CAD build for the part. Positions are in the model's coordinates, mm. Face numbers are marked on the shaded views. Give positions to 0.01 mm unless a question says otherwise; leave off trailing zeros. Order: outer loops, then holes, each group sorted by start corner. A loop starts at its lowest first (then second) coordinate and runs counter-clockwise, first axis right, second up. Notation, with made-up numbers: (-13, -14.75) -> (14, -14.75) arc R28 ccw to (14, 20.25) -> close; hole circle Ø8 at (52.5, 8.5). An arc over 180 degrees is marked (long way). Answer as CSV lines item,"result".
Autodesk Inventor part; units mm, degrees
ref_plane "YZ Plane" through (0, 0, 0) normal (1, 0, 0) x (0, 1, 0)
ref_plane "XZ Plane" through (0, 0, 0) normal (0, 1, 0) x (-1, 0, 0)
ref_plane "XY Plane" through (0, 0, 0) normal (0, 0, 1) x (1, 0, 0)
sketch "Sketch1" plane through (0, 0, 0) normal (0, 0, 1) x (1, 0, 0)
  line L0 (-16, -5) -> (16, -5)
  line L1 (16, -5) -> (16, 5)
  line L2 (16, 5) -> (-16, 5)
  line L3 (-16, 5) -> (-16, -5)
  line L4 (-16, -5) -> (16, 5) construction
  line L5 (16, -5) -> (-16, 5) construction
  point P0 (0, 0)
  dimension "d0" = 32
  dimension "d1" = 10
extrude "Plate1" add sketch "Sketch1" along normal blind 0.5
sketch "Sketch2" plane through (15.5, 5, 0) normal (1, 0, 0) x (0, 1, 0)
  line L0 (-10, 0) -> (0, 0)
  line L1 (0, 0) -> (0, 30)
  line L2 (0, 30) -> (-10, 30)
  line L3 (-10, 30) -> (-10, 0)
edge flange "Flange1" height 30 angle 90 thickness 0.5 bend radius 0.5 thickness toward (1, 0, 0) relief tear relief width 0.5 relief depth 0.25 edges at (16, 0, 0.5) wall of the first edge with corners at (15.5, -5, 0) (15.5, 5, 0) (15.5, 5, 30) (15.5, -5, 30)
bend "Bend1"
corner "Corner1"
sketch "Sketch4" plane through (0, 0, 0.5) normal (0, 0, 1) x (1, 0, 0)
  line L0 (-16, -5) -> (-16, 5)
  point P0 (0, 0)
  point P1 (-12, 0)
  point P2 (-2, 0)
  dimension "d13" = 4
  dimension "d14" = 14
hole "Hole1" at (-12, 0, 0.5) at (-2, 0, 0.5) direction (0, 0, -1) diameter 4 end through all
sketch "Sketch5" plane through (16, -5, 30) normal (1, 0, 0) x (0, 0, -1)
  line L0 (0, 0) -> (0, 10)
  point P0 (30, 5)
  point P1 (4, 5)
  point P2 (14, 5)
  dimension "d22" = 4
  dimension "d23" = 14
hole "Hole2" at (16, 0, 26) at (16, 0, 16) direction (-1, 0, 0) diameter 4 end through all
equation "\"d20\" = Thickness"
equation "\"d29\" = Thickness"
equation "\"d3\" = BendReliefWidth"
equation "\"d4\" = BendReliefDepth"
equation "\"d5\" = MinimumRemnant"
equation "\"d6\" = BendRadius"
equation "\"d9\" = BendRadius"
equation "\"d10\" = CornerReliefSize"
equation "\"d11\" = GapSize"
equation "\"d12\" = JacobiRadiusSize"
equation "\"BendRadius\" = Thickness"
equation "\"BendReliefWidth\" = Thickness"
equation "\"BendReliefDepth\" = 0.5 * Thickness"
equation "\"CornerReliefSize\" = 4 * Thickness"
equation "\"MinimumRemnant\" = 2 * Thickness"
equation "\"TransitionRadius\" = BendRadius"
equation "\"JacobiRadiusSize\" = BendRadius"
equation "\"GapSize\" = Thickness"
equation "\"d2\" = BendRadius"
properties part number "maker-beam-corner"
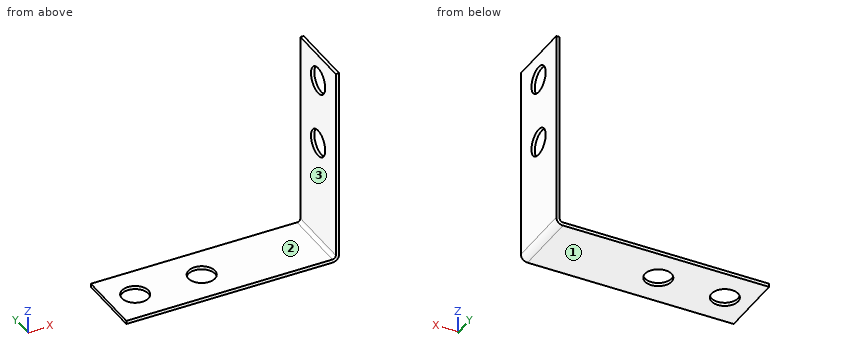
1) Band-saw the part on D-D, the plane y = -1.5. Write the cut outline in (x, z).
Data:
outline,"(-16, 0) -> (-13.32, 0) -> (-13.32, 0.5) -> (-16, 0.5) -> close; (-10.68, 0) -> (-3.32, 0) -> (-3.32, 0.5) -> (-10.68, 0.5) -> close; (-0.68, 0) -> (15, 0) arc R1 ccw to (16, 1) -> (16, 14.68) -> (15.5, 14.68) -> (15.5, 1) arc R0.5 cw to (15, 0.5) -> (-0.68, 0.5) -> close; (15.5, 17.32) -> (16, 17.32) -> (16, 24.68) -> (15.5, 24.68) -> close; (15.5, 27.32) -> (16, 27.32) -> (16, 30) -> (15.5, 30) -> close"
2) Band-saw the part on B-B, the plane z = 16. Write the cut outline in (x, y).
Data:
outline,"(15.5, -5) -> (16, -5) -> (16, -2) -> (15.5, -2) -> close; (15.5, 2) -> (16, 2) -> (16, 5) -> (15.5, 5) -> close"
3) Band-saw the part on A-A, the plane x = -12. Write the cut outline in (y, z).
Data:
outline,"(-5, 0) -> (-2, 0) -> (-2, 0.5) -> (-5, 0.5) -> close; (2, 0) -> (5, 0) -> (5, 0.5) -> (2, 0.5) -> close"
4) Wall check: line 1 along Y through (x, z) = (-12, 0.3); line 2 along Z through (x, y) = (15.8, 0); line 3 along Z through (x, y) = (15.7, 0). Give the ranges that are in metal, low to high. Write a range as [from, to].
Data:
line 1,"y = [-5, -2], [2, 5]"
line 2,"z = [0.4, 14], [18, 24], [28, 30]"
line 3,"z = [0.29, 14], [18, 24], [28, 30]"
5) Band-saw the part on C-C, the plane y = 2.5. Write the cut outline in (x, z).
Data:
outline,"(-16, 0) -> (15, 0) arc R1 ccw to (16, 1) -> (16, 30) -> (15.5, 30) -> (15.5, 1) arc R0.5 cw to (15, 0.5) -> (-16, 0.5) -> close"
6) Pin check, flat tips, straight feed: P1, Ø1, axis at x = 11.5, y = -2, coming from the +Z side; P2, Ø3, axis at y = 0, z = 16, coming from the +X side. Stop position of each tip, or through.
Data:
P1,"stops at z = 0.5"
P2,"passes through"
7) Pull direction Z, two halves, no side cores. Call the marked faces 1, 2 and 3: pulls with the +Z half, pulls with the -Z half, needs draft (parallel to the pull), parting line crosses it, or undercut.
Data:
face 1,"pulls with the -Z half"
face 2,"pulls with the +Z half"
face 3,"needs draft"
